Job drawing, mm, ordinate dimensions from the low corner. One solid piece. A direction names the side the tool comes from. Give positions to 0.01 mm unless a question says otherwise; leave off trailing zeros. Order: outer loops, then holes, each group sorted by start corner. A loop starts at its lowest first (then second) coordinate and runs counter-clockwise, first axis right, second up.
1. Slice it at D-D on y = 18. List the corners of the cut face in (x, z) (1 decimal).
2. Probe line 1 (X direction, y = 12.5, z = 6); line 2 (Z direction, x = 137.5, y = 20.5); line 3 (Y direction, x = 78.5, z = 11). List the from-to ranges inside material, lowest first.
3. Slice it at C-C on z = 13.5. List the corners of the cut face in (x, y).
4. Drop flat-ended pins along their axis: pin 1 Ø8.5 at (y, z) = (13, 7) entering from +X; pin 2 Ø2 at (y, z) = (10.5, 10.5) entering from -X; pin 3 Ø12.5 at (x, y) = (44.5, 16.5) entering from -Z. Give the stop position or say it passes through.
5. Slice it at A-A on x = 75.5. List the corners of the cut face in (y, z), and give its area (3 significant figures).
6. Slice it at B-B on y = 11.75. List the corners of the cut face in (x, z).
7. Which spindle directions (+Z, -Z, +X, -X, +Y, -Y) get a long thin tool onto all of the face, cutting with end or side? Do the marked faces 1, 2 and 3. Say none if no direction does.
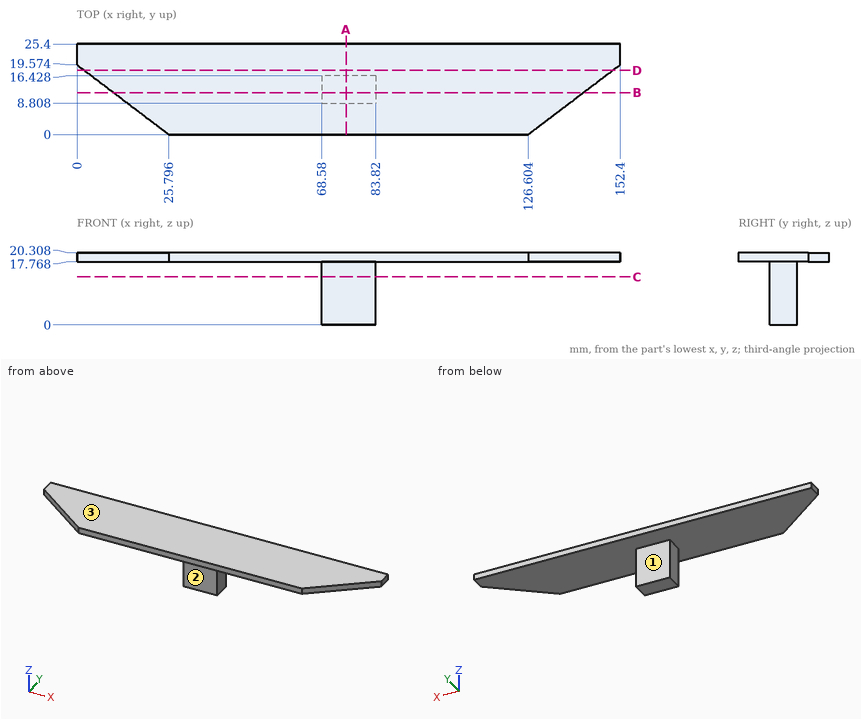
Data:
1. outline: (2.1, 17.8) - (150.3, 17.8) - (150.3, 20.3) - (2.1, 20.3) - close
2. line 1: x = 68.58 to 83.82
2. line 2: z = 17.77 to 20.31
2. line 3: y = 8.81 to 16.43
3. outline: (68.58, 8.81) - (83.82, 8.81) - (83.82, 16.43) - (68.58, 16.43) - close
4. pin 1: stops at x = 83.82
4. pin 2: stops at x = 68.58
4. pin 3: stops at z = 17.77
5. outline: (0, 17.77) - (8.81, 17.77) - (8.81, 0) - (16.43, 0) - (16.43, 17.77) - (25.4, 17.77) - (25.4, 20.31) - (0, 20.31) - close
5. area: 200 mm2
6. outline: (10.31, 17.77) - (68.58, 17.77) - (68.58, 0) - (83.82, 0) - (83.82, 17.77) - (142.09, 17.77) - (142.09, 20.31) - (10.31, 20.31) - close
7. face 1: -Z, +X, -X, +Y
7. face 2: -Z, +X, -X, -Y
7. face 3: +Z, +X, -X, +Y, -Y
